```python
from build123d import *

# Parameters (mm, degrees)
BOSS_EXTRUDE1_DEPTH = 15.875
CUT_EXTRUDE2_REACH  = 49.811
SKETCH3_R           = 2.032
CUT_EXTRUDE3_REACH  = 64.068
SKETCH4_R           = 2.032


with BuildPart() as part:
    # Sketch1 → Boss-Extrude1 (new body)
    with BuildSketch(Plane.XY):
        Polygon((3.175, 3.175), (46.355, 3.175), (46.355, 0), (33.655, 0), (33.655, -12.7), (30.48, -12.7), (30.48, 0), (27.305, 0), (27.305, -12.7), (24.13, -12.7), (24.13, 0), (0, 0), (0, 38.1), (3.175, 38.1), align=None)
    boss_extrude1 = extrude(amount=BOSS_EXTRUDE1_DEPTH)

    # Sketch3 → Cut-Extrude2 (cut, up to next)
    with BuildSketch(Plane.ZY.offset(-24.13), mode=Mode.PRIVATE) as cut_extrude2_sk1:
        with Locations(Location((7.9375, -6.35, 0), (0, 0, 270))):
            Circle(SKETCH3_R)
    cut_extrude2_tool1 = extrude(cut_extrude2_sk1.sketch, amount=-CUT_EXTRUDE2_REACH, mode=Mode.PRIVATE) & part.part
    cut_extrude2 = cut_extrude2_tool1.solids().sort_by_distance((24.13, -6.35, 7.9375))[0]
    add(cut_extrude2, mode=Mode.SUBTRACT)

    # Sketch4 → Cut-Extrude3 (cut, up to next)
    with BuildSketch(Plane.ZY, mode=Mode.PRIVATE) as cut_extrude3_sk1:
        with Locations((7.9375, 31.75)):
            Circle(SKETCH4_R)
    cut_extrude3_tool1 = extrude(cut_extrude3_sk1.sketch, amount=-CUT_EXTRUDE3_REACH, mode=Mode.PRIVATE) & part.part
    cut_extrude3 = cut_extrude3_tool1.solids().sort_by_distance((0, 31.75, 7.9375))[0]
    add(cut_extrude3, mode=Mode.SUBTRACT)

    # Mirror2: Boss-Extrude1, Cut-Extrude2, Cut-Extrude3 across plane
    add(boss_extrude1.mirror(Plane(origin=(46.355, 0, 0), x_dir=(0, 0, 1), z_dir=(1, 0, 0))))
    add(cut_extrude2.mirror(Plane(origin=(46.355, 0, 0), x_dir=(0, 0, 1), z_dir=(1, 0, 0))), mode=Mode.SUBTRACT)
    add(cut_extrude3.mirror(Plane(origin=(46.355, 0, 0), x_dir=(0, 0, 1), z_dir=(1, 0, 0))), mode=Mode.SUBTRACT)


solid = part.part
```
Can you work these out from the model? Positions are in its coordinate system, mm. A direction names the side the tool comes from. Give positions to 0.01 mm unless a question says otherwise; leave off trailing zeros. Loops run counter-clockwise (first coordinate to the right, second up) from the corner with the lowest first, then second, coordinate; pieces in that order, holes last. Notation, with made-up numbers: M 14.25,-28 L 54.25,-28 A31 cw 54.25,-4 Z; hole C -3,89.5 d2. An arc over 180 degrees is marked long. Use one line per item in the form item = value. Start each with the question number.
(1) Please list where these lines run through material, in increasing order: line 1 (X direction, y = -8, z = 11.25) (3 decimals); line 2 (X direction, y = 22, z = 5.5) (3 decimals); line 3 (Y direction, x = 62.5, z = 3) (3 decimals).
(2) I want a section at C-C, the plane y = 31.75. Write out the boundary of the cut face in (x, z) (1 decimal).
(3) I'm going to push flat-ended pins straight in: P1, Ø4, axis at x = 30.5, z = 2, coming from the +Y side (3 decimals); P2, Ø4, axis at y = -8.5, z = 10.5, coming from the +X side; P3, Ø3.5, axis at y = 31.75, z = 7.94, coming from the +X side; P4, Ø1, axis at x = 28, z = 7, coming from the -Y side. Where does each tip first touch, or does it pass through?
(4) On a 3-axis mill with a long thin cutter (end or side, diameter ignored), from which of +Z, -Z, +X, -X, +Y, -Y can I reach the whole of each face in a straight line? I mean faces 4 (the flat face through (80, 0, 8)), 5 (the flat face through (46, 2, 0)), 6 (the flat face through (59.055, -6, 8)), 7 (the flat face through (12, 0, 8)). Say none if no direction works.
(5) I want a section at B-B, the plane y = -6.35. Write out the boundary of the cut face in (x, z) (1 decimal), and give its area (3 significant figures).
(6) I want a section at A-A, the plane y = 21. Write out the boundary of the cut face in (x, z) (3 decimals), and give its area (3 significant figures).
(7) I want a section at D-D, the plane z = 13.75. Write out the boundary of the cut face in (x, y) (3 decimals), and give its area (3 significant figures).
(8) Thinking about a two-plate mould opening in X: for faces 1 (the flat face through (89.535, 21, 8)), 2 (the flat face through (68.58, -5, 6)), 3 (the flat face through (91, 38.1, 8)), which applies, released by +X, released by -X, zero draft, split by the parting line, or undercut?
Worked out:
q1.line_1 = 24.13 to 27.305, 30.48 to 33.655, 59.055 to 62.23, 65.405 to 68.58
q1.line_2 = 0 to 3.175, 89.535 to 92.71
q1.line_3 = 0 to 3.175
q2.outline = M 0,0 L 3.2,0 L 3.2,5.9 L 0,5.9 Z; M 0,10 L 3.2,10 L 3.2,15.9 L 0,15.9 Z; M 89.5,0 L 92.7,0 L 92.7,5.9 L 89.5,5.9 Z; M 89.5,10 L 92.7,10 L 92.7,15.9 L 89.5,15.9 Z
q3.P1 = 3.175
q3.P2 = 68.58
q3.P3 = through
q3.P4 = 0
q4.face_4 = +Z, -Z, +X, -Y
q4.face_5 = -Z, +X, -X, +Y, -Y
q4.face_6 = +Z, -Z, -Y
q4.face_7 = +Z, -Z, -X, -Y
q5.outline = M 24.1,0 L 27.3,0 L 27.3,5.9 L 24.1,5.9 Z; M 24.1,10 L 27.3,10 L 27.3,15.9 L 24.1,15.9 Z; M 30.5,0 L 33.7,0 L 33.7,15.9 L 30.5,15.9 Z; M 59.1,0 L 62.2,0 L 62.2,15.9 L 59.1,15.9 Z; M 65.4,0 L 68.6,0 L 68.6,5.9 L 65.4,5.9 Z; M 65.4,10 L 68.6,10 L 68.6,15.9 L 65.4,15.9 Z
q5.area = 176 mm²
q6.outline = M 0,0 L 3.175,0 L 3.175,15.875 L 0,15.875 Z; M 89.535,0 L 92.71,0 L 92.71,15.875 L 89.535,15.875 Z
q6.area = 101 mm²
q7.outline = M 0,0 L 24.13,0 L 24.13,-12.7 L 27.305,-12.7 L 27.305,0 L 30.48,0 L 30.48,-12.7 L 33.655,-12.7 L 33.655,0 L 59.055,0 L 59.055,-12.7 L 62.23,-12.7 L 62.23,0 L 65.405,0 L 65.405,-12.7 L 68.58,-12.7 L 68.58,0 L 92.71,0 L 92.71,38.1 L 89.535,38.1 L 89.535,3.175 L 3.175,3.175 L 3.175,38.1 L 0,38.1 Z
q7.area = 677 mm²
q8.face_1 = undercut
q8.face_2 = released by +X
q8.face_3 = zero draft
